```python
from build123d import *

# Parameters (mm, degrees)
SKETCH_3_W                         = 193
SKETCH_3_H                         = 140
SM_BASE_FLANGE_1_DEPTH             = 2
SM_EDGE_FLANGE_1_STRIP_W           = 9.4732
SM_EDGE_FLANGE_1_STRIP_H           = 2
SM_EDGE_FLANGE_1_STRIP_CUT_DEPTH   = 140
SM_EDGE_FLANGE_1_STRIP_2_W         = 9.4732
SM_EDGE_FLANGE_1_STRIP_2_H         = 2
SM_EDGE_FLANGE_1_STRIP_CUT_2_DEPTH = 140
SM_EDGE_FLANGE_1_DEPTH             = 140
SM_EDGE_FLANGE_1_BEND_DEPTH        = 140
HOLE_WIZARD_M3_2_D                 = 2.5
HOLE_WIZARD_M3_3_D                 = 2.5
HOLE_WIZARD_M3_3_DEPTH             = 2
HOLE_WIZARD_M3_4_D                 = 2.5
SKETCH_23_W                        = 185
SKETCH_23_H                        = 10
SKETCH_23_W_2                      = 25
SKETCH_23_W_3                      = 70
CUT_EXTRUDE_1_DEPTH                = 10
FILLET_1_R                         = 3
SKETCH_24_W                        = 4
SKETCH_24_H                        = 10
CUT_EXTRUDE_2_DEPTH                = 239.840951263
SKETCH_25_W                        = 4
SKETCH_25_H                        = 10
CUT_EXTRUDE_3_DEPTH                = 10
SKETCH_26_W                        = 4
SKETCH_26_H                        = 10
CUT_EXTRUDE_4_DEPTH                = 10


# Sheet-metal steps are written as plain solids
with BuildPart() as part:
    # ｽｹｯﾁ3 → ﾍﾞｰｽ-ﾌﾗﾝｼﾞ1 (new body)
    with BuildSketch(Plane.XY):
        with Locations((96.5, 70)):
            Rectangle(SKETCH_3_W, SKETCH_3_H)
    extrude(amount=-SM_BASE_FLANGE_1_DEPTH)

    # ｴｯｼﾞ-ﾌﾗﾝｼﾞ1 strip (across the edge) → ｴｯｼﾞ-ﾌﾗﾝｼﾞ1 strip cut (cut)
    with BuildSketch(Plane(origin=(0, 0, -2), x_dir=(1, 0, 0), z_dir=(0, 1, 0))):
        with Locations((-2, -1)):
            Rectangle(SM_EDGE_FLANGE_1_STRIP_W, SM_EDGE_FLANGE_1_STRIP_H)
    extrude(amount=SM_EDGE_FLANGE_1_STRIP_CUT_DEPTH, mode=Mode.SUBTRACT)

    # ｴｯｼﾞ-ﾌﾗﾝｼﾞ1 strip 2 (across the edge) → ｴｯｼﾞ-ﾌﾗﾝｼﾞ1 strip cut 2 (cut)
    with BuildSketch(Plane(origin=(193, 140, -2), x_dir=(-1, 0, 0), z_dir=(0, -1, 0))):
        with Locations((-2, -1)):
            Rectangle(SM_EDGE_FLANGE_1_STRIP_2_W, SM_EDGE_FLANGE_1_STRIP_2_H)
    extrude(amount=SM_EDGE_FLANGE_1_STRIP_CUT_2_DEPTH, mode=Mode.SUBTRACT)

    # ｴｯｼﾞ-ﾌﾗﾝｼﾞ1 section (across the edge) → ｴｯｼﾞ-ﾌﾗﾝｼﾞ1 (add)
    with BuildSketch(Plane(origin=(0, 0, -2), x_dir=(1, 0, 0), z_dir=(0, 1, 0))):
        with BuildLine():
            Line((0, 0.7366), (0, 12))
            Line((0, 12), (2, 12))
            Line((2, 12), (2, 0.7366))
            ThreePointArc((2, 0.7366), (2.215745145, 0.215745145), (2.7366, 0))
            Line((2.7366, 0), (2.7366, -2))
            ThreePointArc((2.7366, -2), (0.801531583, -1.198468417), (0, 0.7366))
        make_face()
    extrude(amount=SM_EDGE_FLANGE_1_DEPTH)

    # ｴｯｼﾞ-ﾌﾗﾝｼﾞ1 section 2 (across the edge) → ｴｯｼﾞ-ﾌﾗﾝｼﾞ1 bend (add)
    with BuildSketch(Plane(origin=(193, 140, -2), x_dir=(-1, 0, 0), z_dir=(0, -1, 0))):
        with BuildLine():
            Line((0, 0.7366), (0, 12))
            Line((0, 12), (2, 12))
            Line((2, 12), (2, 0.7366))
            ThreePointArc((2, 0.7366), (2.215745145, 0.215745145), (2.7366, 0))
            Line((2.7366, 0), (2.7366, -2))
            ThreePointArc((2.7366, -2), (0.801531583, -1.198468417), (0, 0.7366))
        make_face()
    extrude(amount=SM_EDGE_FLANGE_1_BEND_DEPTH)

    # M3 ねじ穴2 (through all)
    with Locations(Plane.XY):
        with Locations((35, 132.5), (35, 15.5), (111.2, 15.5), (111.2, 132.5)):
            Hole(HOLE_WIZARD_M3_2_D / 2)

    # M3 ねじ穴3
    with Locations(Plane.ZY):
        with Locations((-9, 130), (-9, 10)):
            Hole(HOLE_WIZARD_M3_3_D / 2, depth=HOLE_WIZARD_M3_3_DEPTH)

    # M3 ねじ穴4 (through all)
    with Locations(Plane(origin=(193, 0, 0), x_dir=(0, 0, -1), z_dir=(1, 0, 0))):
        with Locations((9, 130), (9, 10)):
            Hole(HOLE_WIZARD_M3_4_D / 2)

    # ｽｹｯﾁ23 → ｶｯﾄ - 押し出し1 (cut)
    with BuildSketch(Plane.XY):
        with Locations((96.5, 5)):
            Rectangle(SKETCH_23_W, SKETCH_23_H)
        with Locations((16.5, 135)):
            Rectangle(SKETCH_23_W_2, SKETCH_23_H)
        with Locations((154, 135)):
            Rectangle(SKETCH_23_W_3, SKETCH_23_H)
    extrude(amount=-CUT_EXTRUDE_1_DEPTH, mode=Mode.SUBTRACT)

    # ﾌｨﾚｯﾄ1
    fillet_1_edges = [part.edges().sort_by_distance(p)[0] for p in [
        (29, 140, -1),
        (119, 140, -1),
    ]]
    fillet(fillet_1_edges, radius=FILLET_1_R)

    # ｽｹｯﾁ24 → ｶｯﾄ - 押し出し2 (cut, through all)
    with BuildSketch(Plane.ZY):
        with Locations((-2, 5)):
            Rectangle(SKETCH_24_W, SKETCH_24_H)
    extrude(amount=-CUT_EXTRUDE_2_DEPTH, mode=Mode.SUBTRACT)

    # ｽｹｯﾁ25 → ｶｯﾄ - 押し出し3 (cut)
    with BuildSketch(Plane.ZY):
        with Locations((-2, 135)):
            Rectangle(SKETCH_25_W, SKETCH_25_H)
    extrude(amount=-CUT_EXTRUDE_3_DEPTH, mode=Mode.SUBTRACT)

    # ｽｹｯﾁ26 → ｶｯﾄ - 押し出し4 (cut)
    with BuildSketch(Plane(origin=(193, 0, 0), x_dir=(0, 0, -1), z_dir=(1, 0, 0))):
        with Locations((2, 135)):
            Rectangle(SKETCH_26_W, SKETCH_26_H)
    extrude(amount=-CUT_EXTRUDE_4_DEPTH, mode=Mode.SUBTRACT)


solid = part.part
```
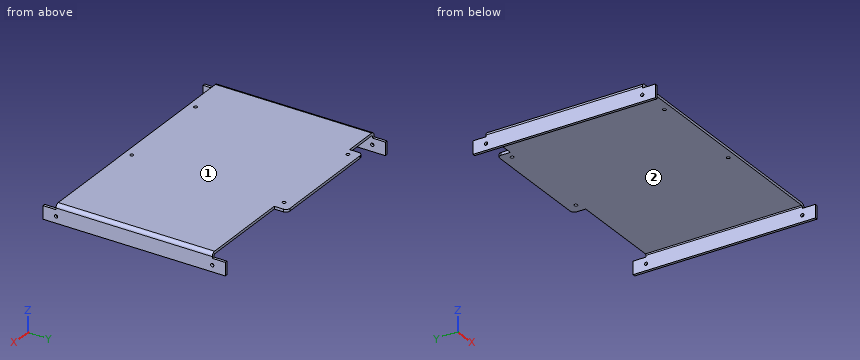
The model under review builds one solid part; all positions refer to its coordinate system, in mm. Face numbers are marked on the shaded views. Round coordinates to 2 decimals unless told otherwise and drop trailing zeros. Order: outer loops, then holes, each group sorted by start corner. A loop starts at its lowest first (then second) coordinate and runs counter-clockwise, first axis right, second up. Notation, with made-up numbers: (51, 88.25) -> (55, 88.25) arc R23 ccw to (55, 113.25) -> close; hole circle Ø5 at (-34, 40). An arc over 180 degrees is marked (long way). Use a Markdown table: item, result.
Q1. For line 1 (Y direction, x = 35, z = -0.9); line 2 (X direction, y = 132.5, z = -1.05); line 3 (Y direction, x = 192.5, z = -9), list the stretches that pass through material, from the lowest coordinate up.
Values:
| item | result |
|---|---|
| line 1 | y = 10 to 14.25, 16.75 to 131.25, 133.75 to 140 |
| line 2 | x = 29 to 33.75, 36.25 to 109.95, 112.45 to 119 |
| line 3 | y = 0 to 8.75, 11.25 to 128.75, 131.25 to 140 |
Q2. We need section A-A on y = 100.5. Write out the cut boundary in (x, z).
Values:
| item | result |
|---|---|
| outline | (0, -14) -> (2, -14) -> (2, -2.74) arc R0.74 cw to (2.74, -2) -> (190.26, -2) arc R0.74 cw to (191, -2.74) -> (191, -14) -> (193, -14) -> (193, -2.74) arc R2.74 ccw to (190.26, 0) -> (2.74, 0) arc R2.74 ccw to (0, -2.74) -> close |
Q3. Mouldability with a two-part tool opening along X and no side actions: class the marked faces 1 and 2 as +X half, -X half, draft (parallel to the pull), parting line (faces both ways), or undercut.
Values:
| item | result |
|---|---|
| face 1 | draft |
| face 2 | undercut |
Q4. Clearance check with flat-ended pins moving along their axes: P1, Ø1, axis at x = 192, y = 137, coming from the +Z side; P2, Ø1.6, axis at y = 132, z = -1.5, coming from the -X side; P3, Ø3, axis at x = 111.2, y = 132.5, coming from the -Z side. State where each tip first meets the part, or that it passes through.
Values:
| item | result |
|---|---|
| P1 | stops at z = -4 |
| P2 | stops at x = 29 |
| P3 | stops at z = -2 |
Q5. We need section C-C on x = 101.5. Write out the cut boundary in (y, z), then the cut area to 3 significant figures.
Values:
| item | result |
|---|---|
| outline | (10, -2) -> (140, -2) -> (140, 0) -> (10, 0) -> close |
| area | 260 mm^2 |
Q6. We need section B-B on x = 137. Write out the cut boundary in (y, z).
Values:
| item | result |
|---|---|
| outline | (10, -2) -> (130, -2) -> (130, 0) -> (10, 0) -> close |
